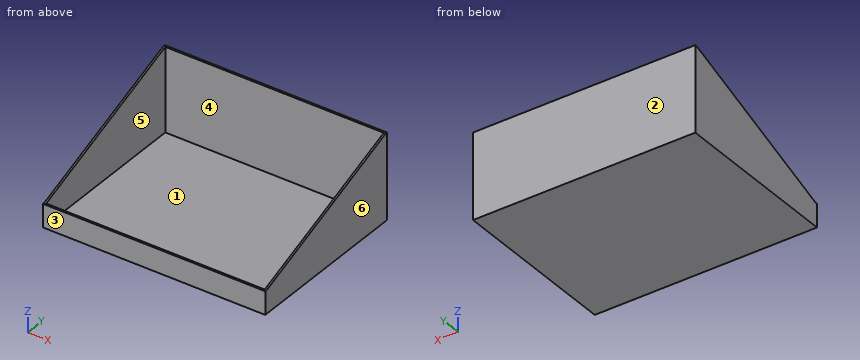
from build123d import *

# Parameters (mm, degrees)
F0_W     = 480
F0_H     = 185
F1_DEPTH = 370
F3_DEPTH = 480
F5_W     = 472
F5_H     = 362
F6_DEPTH = 181


with BuildPart() as f1:
    # F0 (on Front) → F1 (new body)
    with BuildSketch(Plane.XZ):
        with Locations((-240, 92.5)):
            Rectangle(F0_W, F0_H)
    extrude(amount=-F1_DEPTH)

    # F2 (on Right) → F3 (cut, through all)
    with BuildSketch(Plane.YZ):
        Polygon((0, 50), (4, 50), (366, 185), (0, 185), align=None)
    extrude(amount=-F3_DEPTH, mode=Mode.SUBTRACT)

    # F5 (on plane+point) → F6 (cut)
    with BuildSketch(Plane.XY.offset(185)):
        with Locations((-240, 185)):
            Rectangle(F5_W, F5_H)
    extrude(amount=-F6_DEPTH, mode=Mode.SUBTRACT)


solid = f1.part
Input: part model. Units: mm. Frame: model coordinates. Face numbers are marked on the shaded views. A direction names the side the tool comes from. Give positions to 0.01 mm unless a question says otherwise; leave off trailing zeros. Order: outer loops, then holes, each group sorted by start corner. A loop starts at its lowest first (then second) coordinate and runs counter-clockwise, first axis right, second up. Notation, with made-up numbers: (2.5, -35.75) -> (55.5, -35.75) arc R24 ccw to (55.5, -11.75) -> close; hole circle Ø8 at (19.5, 10). An arc over 180 degrees is marked (long way). Use one line per item in the form item = value.
1) Reachability of the marked faces 5 and 6 from +Z, -Z, +X, -X, +Y, -Y: full face, straight path, thin tool, end or side. Return the list, or none.
Response values:
face_5 = +Z
face_6 = +Z, -Z, +X, +Y, -Y
2) Mould query, pull axis Y, two halves, no side actions, for the marked faces 1, 2, 3 and 4. Classes: pulls with the +Y half, pulls with the -Y half, needs draft (parallel to the pull), parting line crosses it, or undercut.
Response values:
face_1 = undercut
face_2 = pulls with the +Y half
face_3 = pulls with the -Y half
face_4 = undercut
3) Line query: probe 1 along X at (y, z) = (238.5, 135); probe 2 along Y at (x, z) = (-169.5, 10); probe 3 along Y at (x, z) = (-22, 87). Output: solid intervals per line, ascending.
Response values:
probe_1 = -480 to -476, -4 to 0
probe_2 = 0 to 4, 366 to 370
probe_3 = 366 to 370
4) Section A-A, the plane x = -195.5. Return loops of the section in (y, z), and give its area (3 significant figures).
Response values:
outline = (0, 0) -> (370, 0) -> (370, 185) -> (366, 185) -> (366, 4) -> (4, 4) -> (4, 50) -> (0, 50) -> close
area = 2,390 mm^2
5) First-contact query: pin 1 Ø10 at (x, y) = (-190, 218.5) entering from +Z; pin 2 Ø3 at (x, y) = (-163.5, 1.5) entering from +Z. Flat tips, straight axial feed; report the tip coordinate or a pass-through.
Response values:
pin_1 = 4
pin_2 = 50
6) Section C-C, the plane z = 144.5. Return loops of the section in (x, y), and give its area (3 significant figures).
Response values:
outline = (-480, 257.4) -> (-476, 257.4) -> (-476, 366) -> (-4, 366) -> (-4, 257.4) -> (0, 257.4) -> (0, 370) -> (-480, 370) -> close
area = 2,790 mm^2
7) Section B-B, the plane z = 33. Return loops of the section in (x, y), and give its area (3 significant figures).
Response values:
outline = (-480, 0) -> (0, 0) -> (0, 370) -> (-480, 370) -> close; hole (-476, 4) -> (-4, 4) -> (-4, 366) -> (-476, 366) -> close
area = 6,740 mm^2
